The listing builds one solid part. Answer for the finished solid, in the listing's coordinates (mm). Round coordinates to 2 decimals unless told otherwise and drop trailing zeros. Order: outer loops, then holes, each group sorted by start corner. A loop starts at its lowest first (then second) coordinate and runs counter-clockwise, first axis right, second up. Notation, with made-up numbers: M 33.5,-27 L 81.5,-27 A21 cw 81.5,7 Z; hole C -25,-22 d6. An arc over 180 degrees is marked long. Put each result on its own line as item: value. Start each with the question number.
1. This flat-tipped pin is pushed along its axis until it touches: pin 1 Ø2 at (x, y) = (-11.5, -1.5) entering from +Z. Where does it stop, or does it pass through?
2. The part is cut by section B-B (x = -1.5). Give the vertices of the cut face in (y, z).
3. Consider line 1 (Z direction, x = -58.5, y = 1.35); line 2 (X direction, y = -0.7, z = 15.5); line 3 (X direction, y = -0.5, z = 0). Determine where each line is inside the solid, lowest interval first.
4. The part is cut by section A-A (z = -10.5). Give the vertices of the cut face in (x, y).
5. The part is cut by section C-C (y = 1.3). Count the separate pieces of the cut face and the enclosed holes in it, then the cut area to 3 significant figures.
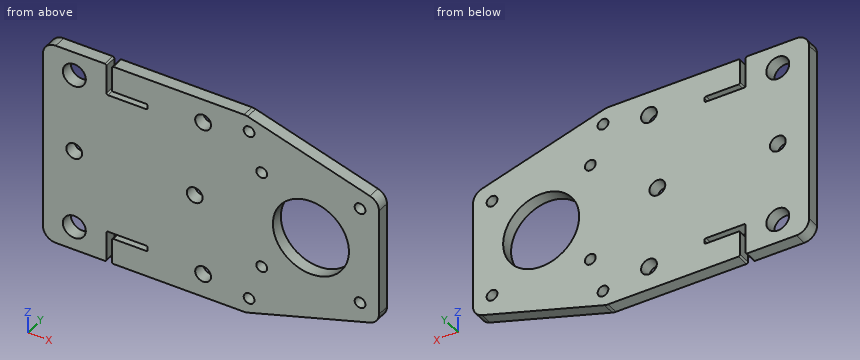
from build123d import *

# Parameters (mm, degrees)
SKETCH1_R           = 12
BOSS_EXTRUDE1_DEPTH = 2
SKETCH2_R           = 1.7
CUT_EXTRUDE1_DEPTH  = 91.622844802
SKETCH3_R           = 2.5
SKETCH3_R_2         = 3.625
CUT_EXTRUDE2_DEPTH  = 91.622844802
CUT_EXTRUDE3_DEPTH  = 91.622844802
FILLET1_R           = 4
FILLET2_R           = 0.5


with BuildPart() as part:
    # Sketch1 → Boss-Extrude1 (new, symmetric)
    with BuildSketch(Plane(origin=(0, 0, 0), x_dir=(1, 0, 0), z_dir=(0, 1, 0))):
        Polygon((21.5, 20), (21.5, -20), (-20.5, -32.5), (-84.5, -32.5), (-84.5, 32.5), (-20.5, 32.5), align=None)
        with Locations(Location((0, 0, 0), (0, 0, 270))):
            Circle(SKETCH1_R, mode=Mode.SUBTRACT)
    extrude(amount=BOSS_EXTRUDE1_DEPTH, both=True)

    # Sketch2 → Cut-Extrude1 (cut, through all)
    with BuildSketch(Plane(origin=(0, 2, 0), x_dir=(1, 0, 0), z_dir=(0, 1, 0))):
        with Locations(Location((15.5, 15.5, 0), (0, 0, 270))):
            Circle(SKETCH2_R)
        with Locations(Location((-15.5, 15.5, 0), (0, 0, 270))):
            Circle(SKETCH2_R)
        with Locations(Location((-15.5, -15.5, 0), (0, 0, 270))):
            Circle(SKETCH2_R)
        with Locations(Location((15.5, -15.5, 0), (0, 0, 270))):
            Circle(SKETCH2_R)
        with Locations(Location((-19.5, 27.5, 0), (0, 0, 270))):
            Circle(SKETCH2_R)
        with Locations(Location((-19.5, -27.5, 0), (0, 0, 270))):
            Circle(SKETCH2_R)
    extrude(amount=-CUT_EXTRUDE1_DEPTH, mode=Mode.SUBTRACT)

    # Sketch3 → Cut-Extrude2 (cut, through all)
    with BuildSketch(Plane(origin=(0, 2, 0), x_dir=(1, 0, 0), z_dir=(0, 1, 0))):
        with Locations(Location((-74.65, 0, 0), (0, 0, 270))):
            Circle(SKETCH3_R)
        with Locations(Location((-36.65, 0, 0), (0, 0, 270))):
            Circle(SKETCH3_R)
        with Locations(Location((-34, 25, 0), (0, 0, 270))):
            Circle(SKETCH3_R)
        with Locations(Location((-34, -25, 0), (0, 0, 270))):
            Circle(SKETCH3_R)
        with Locations(Location((-74.625, 25, 0), (0, 0, 270))):
            Circle(SKETCH3_R_2)
        with Locations(Location((-74.625, -25, 0), (0, 0, 270))):
            Circle(SKETCH3_R_2)
    extrude(amount=-CUT_EXTRUDE2_DEPTH, mode=Mode.SUBTRACT)

    # Sketch4 → Cut-Extrude3 (cut, through all)
    with BuildSketch(Plane(origin=(0, 2, 0), x_dir=(1, 0, 0), z_dir=(0, 1, 0))):
        Polygon((-64.5, 32.5), (-64.5, 22.5), (-51.5, 22.5), (-51.5, 24.25), (-62.75, 24.25), (-62.75, 32.5), align=None)
        Polygon((-62.75, -24.25), (-62.75, -32.5), (-64.5, -32.5), (-64.5, -22.5), (-51.5, -22.5), (-51.5, -24.25), align=None)
    extrude(amount=-CUT_EXTRUDE3_DEPTH, mode=Mode.SUBTRACT)

    # Fillet1
    fillet1_edges = [part.edges().sort_by_distance(p)[0] for p in [
        (-20.5, 0, 32.5),
        (-84.5, 0, 32.5),
        (-84.5, 0, -32.5),
        (-20.5, 0, -32.5),
        (21.5, 0, -20),
        (21.5, 0, 20),
    ]]
    fillet(fillet1_edges, radius=FILLET1_R)

    # Fillet2
    fillet2_edges = [part.edges().sort_by_distance(p)[0] for p in [
        (-62.75, 0, 24.25),
        (-62.75, 0, 32.5),
        (-64.5, 0, 32.5),
        (-64.5, 0, 22.5),
        (-51.5, 0, 22.5),
        (-64.5, 0, -32.5),
        (-62.75, 0, -32.5),
        (-62.75, 0, -24.25),
        (-51.5, 0, -24.25),
        (-51.5, 0, -22.5),
        (-64.5, 0, -22.5),
        (-51.5, 0, 24.25),
    ]]
    fillet(fillet2_edges, radius=FILLET2_R)


solid = part.part
Resolved:
1. pin 1: z = 30.12
2. outline: M -2,-26.85 L 2,-26.85 L 2,-11.91 L -2,-11.91 Z; M -2,11.91 L 2,11.91 L 2,26.85 L -2,26.85 Z
3. line 1: -32.5 to -24.25, -22.5 to 22.5, 24.25 to 32.5
3. line 2: -84.5 to -17.2, -13.8 to 13.8, 17.2 to 21.5
3. line 3: -84.5 to -77.15, -72.15 to -39.15, -34.15 to -12, 12 to 21.5
4. outline: M -84.5,-2 L -5.81,-2 L -5.81,2 L -84.5,2 Z; M 5.81,-2 L 21.5,-2 L 21.5,2 L 5.81,2 Z
5. separate pieces: 1
5. enclosed holes: 13
5. area: 5,610 mm2
